Read the model definition and answer for the solid it produces. Units are mm, in the model's axes. Give positions to 0.01 mm unless a question says otherwise; leave off trailing zeros. Loops run counter-clockwise (first coordinate to the right, second up) from the corner with the lowest first, then second, coordinate; pieces in that order, holes last. Notation, with made-up numbers: (84, 72.25) - (120, 72.25) arc R26 ccw to (120, 107.25) - close; hole circle Ø7 at (36.5, -29.75). An arc over 180 degrees is marked (long way). Write each question's results on one line, items separated by ' | '. Start each with the question number.
Q1. Find the intervals of material crossed by line 1 (Z direction, x = 29.5, y = -83.5), in increasing order. Write a range as from..to.
Q2. The part is cut by section C-C, the plane x = 106. Write down the section's boundary in (y, z), plus the area to 3 significant figures.
Q3. Given pin 1 (3 mm diameter, centred on y = -127, z = -2.5, fed in from -X); pin 2 (6 mm diameter, centred on x = 37.5, y = -188, fed in from -Z); pin 3 (1.5 mm diameter, centred on y = -227, z = -3.5, fed in from +X), each flat-ended and moving along its own axis, determine where each tip first touches the part or whether it passes through.
Q4. The part is cut by section A-A, the plane z = 4.75. Write down the section's boundary in (x, y), plus the area to 3 significant figures.
```python
from build123d import *

# Parameters (mm, degrees)
F0_W     = 330.2
F0_H     = 5.08
F1_DEPTH = 50.8
F3_DEPTH = 25.4
F5_DEPTH = 101.6
F7_DEPTH = 25.4
F9_DEPTH = 50.8
F10_R    = 5.07999


# Not quite as in the source:
# - a fillet or chamfer is up to 0.001 mm smaller than in the source, because OpenCascade refuses the exact size


with BuildPart() as f1:
    # F0 (on Front) → F1 (new body)
    with BuildSketch(Plane.XZ):
        with Locations((5.0749575138, -2.54)):
            Rectangle(F0_W, F0_H)
    extrude(amount=F1_DEPTH)

    # F2 (on face) → F3 (join)
    with BuildSketch(Plane.XZ.offset(50.8)):
        Polygon((170.1749575138, -5.08), (170.1749575138, 0), (-160.0250424862, 0), (-160.0250424862, -5.08), (154.9349575138, -5.08), align=None)
        Polygon((170.1749575138, 12.7), (170.1749575138, 0), (170.1749575138, -5.08), (154.9349575138, -5.08), (154.9349575138, -10.16), (175.2549575138, -10.16), (175.2549575138, 12.7), align=None)
    extrude(amount=F3_DEPTH)

    # F4 (on face) → F5 (join)
    with BuildSketch(Plane.XZ.offset(76.2)):
        Polygon((170.1749575138, 0), (-160.0250424862, 0), (-160.0250424862, -5.08), (154.9349575138, -5.08), (170.1749575138, -5.08), align=None)
    extrude(amount=F5_DEPTH)

    # F6 (on face) → F7 (join)
    with BuildSketch(Plane.XZ.offset(177.8)):
        Polygon((170.1749575138, -5.08), (170.1749575138, 0), (-160.0250424862, 0), (-160.0250424862, -5.08), (154.9349575138, -5.08), align=None)
        Polygon((170.1749575138, 12.7), (170.1749575138, 0), (170.1749575138, -5.08), (154.9349575138, -5.08), (154.9349575138, -10.16), (175.2549575138, -10.16), (175.2549575138, 12.7), align=None)
    extrude(amount=F7_DEPTH)

    # F8 (on face) → F9 (join)
    with BuildSketch(Plane.XZ.offset(203.2)):
        Polygon((170.1749575138, 0), (-160.0250424862, 0), (-160.0250424862, -5.08), (154.9349575138, -5.08), (170.1749575138, -5.08), align=None)
    extrude(amount=F9_DEPTH)

    # F10 (radius 5.08 in the source; OpenCascade refuses exactly that, so slightly less here)
    f10_edges = [f1.edges().sort_by_distance(p)[0] for p in [
        (-160.025042, -127, -5.08),
    ]]
    fillet(f10_edges, radius=F10_R)


solid = f1.part
```
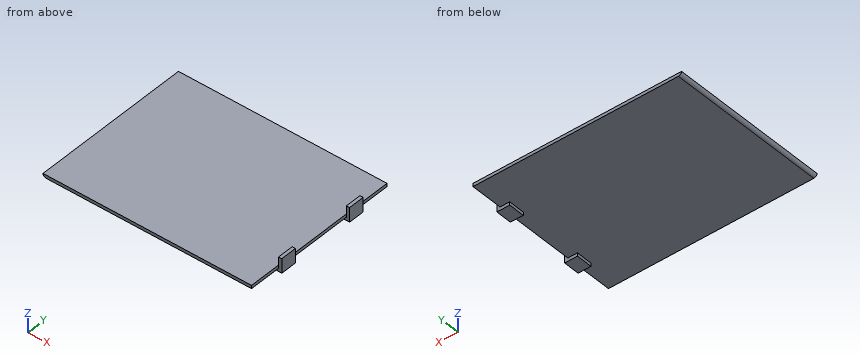
Check sheet entries:
1) line 1: z = -5.08..0
2) outline: (-254, -5.08) - (0, -5.08) - (0, 0) - (-254, 0) - close | area: 1,290 mm^2
3) pin 1: stops at x = -159.93 | pin 2: stops at z = -5.08 | pin 3: stops at x = 170.17
4) outline: (170.17, -203.2) - (175.25, -203.2) - (175.25, -177.8) - (170.17, -177.8) - close; (170.17, -76.2) - (175.25, -76.2) - (175.25, -50.8) - (170.17, -50.8) - close | area: 258 mm^2
